Here's how the part is built. I have some questions about the finished solid (model axes, mm). Round coordinates to 2 decimals unless told otherwise and drop trailing zeros. Write each loop counter-clockwise with the first axis right and the second up, starting at its lowest first coordinate (ties: lowest second). Pieces come first, ordered by that corner, then holes. Notation, with made-up numbers: (32, 51) -> (70, 51) arc R24 cw to (70, 87) -> close; hole circle Ø2 at (60, 39). An arc over 180 degrees is marked (long way). Answer in a Markdown table with one row per item.
from build123d import *

# Parameters (mm, degrees)
F0_R     = 11
F1_DEPTH = 7
F2_R     = 4
F3_DEPTH = 25
F4_R     = 0.3


with BuildPart() as f1:
    # F0 (on Front) → F1 (new body)
    with BuildSketch(Plane.XZ):
        Circle(F0_R)
    extrude(amount=F1_DEPTH)

    # F2 (on face) → F3 (cut)
    with BuildSketch(Plane.XZ.offset(7)):
        Circle(F2_R)
    extrude(amount=-F3_DEPTH, mode=Mode.SUBTRACT)

    # F4
    f4_edges = [f1.edges().sort_by_distance(p)[0] for p in [
        (-11, -7, 0),
        (-11, 0, 0),
        (-4, 0, 0),
        (-4, -7, 0),
    ]]
    fillet(f4_edges, radius=F4_R)


solid = f1.part
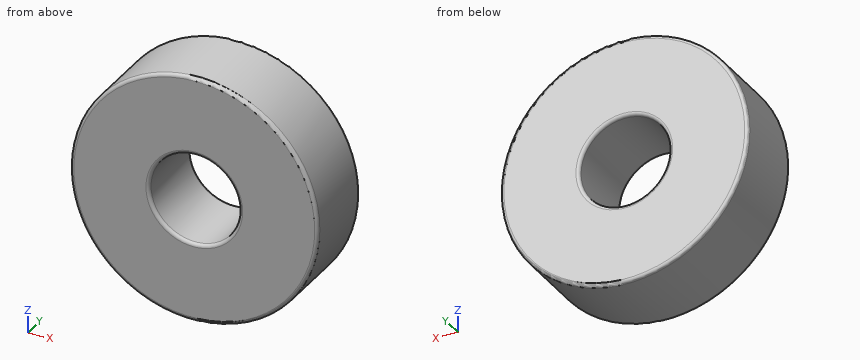
1) I want a section at C-C, the plane y = -2. List the corners of the cut face in (x, z) for me, and give its area (3 significant figures).
Response:
| item | result |
|---|---|
| outline | circle Ø22 at (0, 0); hole circle Ø8 at (0, 0) |
| area | 330 mm^2 |
2) I want a section at B-B, the plane x = 0. List the corners of the cut face in (y, z) for me.
Response:
| item | result |
|---|---|
| outline | (-7, -10.7) arc R0.3 ccw to (-6.7, -11) -> (-0.3, -11) arc R0.3 ccw to (0, -10.7) -> (0, -4.3) arc R0.3 ccw to (-0.3, -4) -> (-6.7, -4) arc R0.3 ccw to (-7, -4.3) -> close; (-7, 4.3) arc R0.3 ccw to (-6.7, 4) -> (-0.3, 4) arc R0.3 ccw to (0, 4.3) -> (0, 10.7) arc R0.3 ccw to (-0.3, 11) -> (-6.7, 11) arc R0.3 ccw to (-7, 10.7) -> close |
3) For pin 1 (1 mm diameter, centred on x = 4, y = -5, fed in from -Z); pin 2 (1 mm diameter, centred on y = -5, z = -6, fed in from +X); pin 3 (6.5 mm diameter, centred on x = 0, z = 0, fed in from -Y), each with a flat end and sliding along its axis, tell me the tip position at first contact or that it passes through.
Response:
| item | result |
|---|---|
| pin 1 | stops at z = -10.43 |
| pin 2 | stops at x = 9.53 |
| pin 3 | passes through |
4) I need wall thicknesses on line 1 (Z direction, x = 0, y = -4.75); line 2 (Y direction, x = 3, z = -3); line 3 (X direction, y = -1.75, z = 0.75). Which ranges of each line are inside material? Lowest first, please. Write a range as [from, to].
Response:
| item | result |
|---|---|
| line 1 | z = [-11, -4], [4, 11] |
| line 2 | y = [-6.99, -0.01] |
| line 3 | x = [-10.97, -3.93], [3.93, 10.97] |
5) I want a section at A-A, the plane z = 0. List the corners of the cut face in (x, y) for me, and give its area (3 significant figures).
Response:
| item | result |
|---|---|
| outline | (-11, -6.7) arc R0.3 ccw to (-10.7, -7) -> (-4.3, -7) arc R0.3 ccw to (-4, -6.7) -> (-4, -0.3) arc R0.3 ccw to (-4.3, 0) -> (-10.7, 0) arc R0.3 ccw to (-11, -0.3) -> close; (4, -6.7) arc R0.3 ccw to (4.3, -7) -> (10.7, -7) arc R0.3 ccw to (11, -6.7) -> (11, -0.3) arc R0.3 ccw to (10.7, 0) -> (4.3, 0) arc R0.3 ccw to (4, -0.3) -> close |
| area | 97.8 mm^2 |
